Geometry: final body of the model. Coordinates: model frame, mm. A direction names the side the tool comes from. Round coordinates to 2 decimals unless told otherwise and drop trailing zeros. Loops run counter-clockwise (first coordinate to the right, second up) from the corner with the lowest first, then second, coordinate; pieces in that order, holes last. Notation, with made-up numbers: (-4, 53.25) - (20, 53.25) arc R33 cw to (20, 92.25) - close; hole circle Ø11 at (88.5, 57.25). An arc over 180 degrees is marked (long way). Return JSON: item names as keys, results as strings. Group by question number.
1. Material intervals for probe 1 along Y at (x, z) = (0, 2.4); probe 2 along Y at (x, z) = (0, 0.7); probe 3 along Y at (x, z) = (-4.5, 0.75), sorted ascending.
2. Draft query along X for faces 1 (the face through (-0.098, -8.256, 1.572)), 2 (the face through (-1.5, 8, 2)), 3 (the face through (0, 6, 1)), 4 (the face through (-4, 7, 2)). Return one class per face: +X half, -X half, draft (parallel to the pull), parting line (faces both ways), or undercut.
3. Section A-A on x = 0. Return loops of the section in (y, z), and give its area (3 significant figures).
4. First-contact query: pin 1 Ø1 at (x, z) = (3, 1) entering from -Y; pin 2 Ø0.9 at (x, z) = (-5, 1) entering from +Y; pin 3 Ø0.8 at (x, z) = (0.5, 2) entering from -Y. Flat tips, straight axial feed; report the tip coordinate or a pass-through.
5. Section D-D on z = 2.65. Return loops of the section in (x, y).
6. Set-up query: faces 5 (the face through (-4, -7, 2)), 6 (the face through (1.5, 8, 2)), 7 (the face through (6, 0, 1)), 8 (the face through (-5.25, 0, 2)). Return all of +Z, -Z, +X, -X, +Y, -Y with unobstructed straight access to the full face (end or side cutting, diameter ignored); none if empty.
7. Section B-B on y = 1. Return loops of the section in (x, z).
from build123d import *

# Parameters (mm, degrees)
SKETCH_1_W          = 14
SKETCH_1_H          = 14
SKETCH_1_W_2        = 12
SKETCH_1_H_2        = 12
EXTRUDE_1_DEPTH     = 1.5
SKETCH_2_W          = 3
SKETCH_2_H          = 1.5
EXTRUDE_2_DEPTH     = 3.5
SKETCH_3_R          = 0.75
CUT_EXTRUDE_1_DEPTH = 3.5
CUT_EXTRUDE_2_DEPTH = 3.5
EXTRUDE_START       = 1.6
SKETCH_6_R          = 0.75
SKETCH_6_W          = 10.5
SKETCH_6_H          = 10.5
EXTRUDE_3_DEPTH     = 1.6


with BuildPart() as part:
    # 草图1 → 凸台-拉伸1 (new body)
    with BuildSketch(Plane.XY):
        Rectangle(SKETCH_1_W, SKETCH_1_H)
        Rectangle(SKETCH_1_W_2, SKETCH_1_H_2, mode=Mode.SUBTRACT)
    extrude(amount=EXTRUDE_1_DEPTH)

    # 草图2 → 凸台-拉伸2 (add)
    with BuildSketch(Plane.XZ.offset(7)):
        with Locations((0, 0.75)):
            Rectangle(SKETCH_2_W, SKETCH_2_H)
    extrude_2 = extrude(amount=EXTRUDE_2_DEPTH)

    # 草图3 → 切除-拉伸1 (cut)
    with BuildSketch(Plane.XY.offset(1.5)):
        with Locations((0, -9)):
            Circle(SKETCH_3_R)
    cut_extrude_1 = extrude(amount=-CUT_EXTRUDE_1_DEPTH, mode=Mode.SUBTRACT)

    # 草图3<3> → 切除-拉伸2 (cut)
    with BuildSketch(Plane.XY.offset(1.5)):
        with BuildLine():
            ThreePointArc((0, -10.5), (-1.060660172, -10.060660172), (-1.5, -9))
            Line((-1.5, -9), (-1.5, -10.5))
            Line((-1.5, -10.5), (0, -10.5))
        make_face()
        with BuildLine():
            Line((1.5, -10.5), (1.5, -9))
            ThreePointArc((1.5, -9), (1.060660172, -10.060660172), (0, -10.5))
            Line((0, -10.5), (1.5, -10.5))
        make_face()
    cut_extrude_2 = extrude(amount=-CUT_EXTRUDE_2_DEPTH, mode=Mode.SUBTRACT)

    # 镜向1: 凸台-拉伸2, 切除-拉伸1, 切除-拉伸2 across plane
    add(extrude_2.mirror(Plane.ZX))
    add(cut_extrude_1.mirror(Plane.ZX), mode=Mode.SUBTRACT)
    add(cut_extrude_2.mirror(Plane.ZX), mode=Mode.SUBTRACT)

    # 草图6 → 凸台-拉伸3 (add)
    with BuildSketch(Plane.XY.offset(1.5).offset(EXTRUDE_START)):
        with BuildLine():
            Line((-1.5, -9), (-1.5, -7))
            Line((-1.5, -7), (-7, -7))
            Line((-7, -7), (-7, 7))
            Line((-7, 7), (-1.5, 7))
            Line((-1.5, 7), (-1.5, 9))
            ThreePointArc((-1.5, 9), (0, 10.5), (1.5, 9))
            Line((1.5, 9), (1.5, 7))
            Line((1.5, 7), (7, 7))
            Line((7, 7), (7, -7))
            Line((7, -7), (1.5, -7))
            Line((1.5, -7), (1.5, -9))
            ThreePointArc((1.5, -9), (0, -10.5), (-1.5, -9))
        make_face()
        with Locations((0, 9)):
            Circle(SKETCH_6_R, mode=Mode.SUBTRACT)
        with Locations((0, -9)):
            Circle(SKETCH_6_R, mode=Mode.SUBTRACT)
        Rectangle(SKETCH_6_W, SKETCH_6_H, mode=Mode.SUBTRACT)
    extrude(amount=-EXTRUDE_3_DEPTH)


solid = part.part
Taken from the geometry:
{
 "1": {"probe 1": "-10.5 to -9.75, -8.25 to -5.25, 5.25 to 8.25, 9.75 to 10.5", "probe 2": "-10.5 to -9.75, -8.25 to -6, 6 to 8.25, 9.75 to 10.5", "probe 3": "-7 to -6, 6 to 7"},
 "2": {"face 1": "undercut", "face 2": "-X half", "face 3": "undercut", "face 4": "draft"},
 "3": {"outline": "(-10.5, 0) - (-9.75, 0) - (-9.75, 3.1) - (-10.5, 3.1) - close; (-8.25, 0) - (-6, 0) - (-6, 1.5) - (-5.25, 1.5) - (-5.25, 3.1) - (-8.25, 3.1) - close; (5.25, 1.5) - (6, 1.5) - (6, 0) - (8.25, 0) - (8.25, 3.1) - (5.25, 3.1) - close; (9.75, 0) - (10.5, 0) - (10.5, 3.1) - (9.75, 3.1) - close", "area": "21.0 mm2"},
 "4": {"pin 1": "y = -7", "pin 2": "y = 7", "pin 3": "y = -10.5"},
 "5": {"outline": "(-7, -7) - (-1.5, -7) - (-1.5, -9) arc R1.5 ccw to (1.5, -9) - (1.5, -7) - (7, -7) - (7, 7) - (1.5, 7) - (1.5, 9) arc R1.5 ccw to (-1.5, 9) - (-1.5, 7) - (-7, 7) - close; hole (-5.25, -5.25) - (5.25, -5.25) - (5.25, 5.25) - (-5.25, 5.25) - close; hole circle Ø1.5 at (0, -9); hole circle Ø1.5 at (0, 9)"},
 "6": {"face 5": "+Z, -Z, -X, -Y", "face 6": "+Z, -Z, +X, +Y", "face 7": "-Z", "face 8": "+Z, -Z"},
 "7": {"outline": "(-7, 0) - (-6, 0) - (-6, 1.5) - (-5.25, 1.5) - (-5.25, 3.1) - (-7, 3.1) - close; (5.25, 1.5) - (6, 1.5) - (6, 0) - (7, 0) - (7, 3.1) - (5.25, 3.1) - close"}
}
